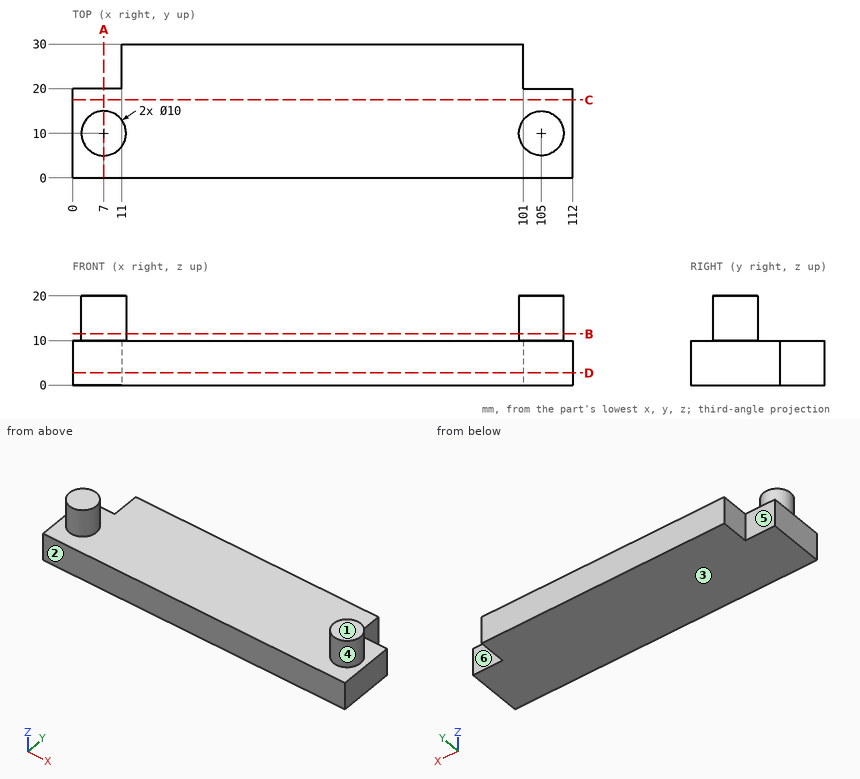
Answer from the drawing. Dimensions are ordinates in mm from the lowest x, y and z of the part. A direction names the side the tool comes from. Give positions to 0.01 mm unless a question says otherwise; leave off trailing zeros. Order: outer loops, then holes, each group sorted by start corner. A loop starts at its lowest first (then second) coordinate and runs counter-clockwise, first axis right, second up. Notation, with made-up numbers: (62, 69) - (102, 69) arc R11 ccw to (102, 86) - close; hole circle Ø8 at (28.5, -37.75). An arc over 180 degrees is marked (long way). Use one line per item in the form item = value.
1) Find section B-B on z = 11.5. Determine the outline of the cut face in (x, y).
Verdict:
outline = circle Ø10 at (7, 10); circle Ø10 at (105, 10)
2) Each of these flat-tipped pins is pushed along its axis until it touches: pin 1 (5 mm diameter, centred on y = 27, z = 7, fed in from +X); pin 2 (3 mm diameter, centred on x = 93, y = 12, fed in from -Z); pin 3 (3 mm diameter, centred on x = 93, y = 15.5, fed in from +Z); pin 4 (8 mm diameter, centred on x = 108, z = 4.5, fed in from +Y). Where does it stop, or does it pass through?
Verdict:
pin_1 = 101
pin_2 = 0
pin_3 = 10
pin_4 = 20
3) Find section D-D on z = 2.75. Determine the outline of the cut face in (x, y).
Verdict:
outline = (0, 0) - (112, 0) - (112, 20) - (101, 20) - (101, 30) - (11, 30) - (11, 20) - (0, 20) - close
4) Find section A-A on x = 7. Determine the outline of the cut face in (y, z), and give its area (3 significant figures).
Verdict:
outline = (0, 0) - (20, 0) - (20, 10) - (15, 10) - (15, 20) - (5, 20) - (5, 10) - (0, 10) - close
area = 300 mm^2
5) The mould has two halves that part along Z. Classify the marked faces 1, 2 and 3: released by +Z, released by -Z, zero draft, split by the parting line, or undercut.
Verdict:
face_1 = released by +Z
face_2 = zero draft
face_3 = released by -Z
6) Consider probe 1 along Z at (x, y) = (92, 2.5); probe 2 along X at (y, z) = (7, 12.5); probe 3 along X at (y, z) = (20.5, 6.5). Determine where each line is inside the solid, lowest interval first. Write a range as [from, to].
Verdict:
probe_1 = [0, 10]
probe_2 = [3, 11], [101, 109]
probe_3 = [11, 101]
7) For the marked faces 4, 5 and 6, determine the directions among +Z, -Z, +X, -X, +Y, -Y from which every point of the face is accessible in a straight line to the end or side of a thin tool.
Verdict:
face_4 = +Z
face_5 = +Z, -Z, -X, +Y
face_6 = +Z, -Z, +X, +Y
8) Find section C-C on y = 17.5. Determine the outline of the cut face in (x, z).
Verdict:
outline = (0, 0) - (112, 0) - (112, 10) - (0, 10) - close
